```python
from build123d import *

# Parameters (mm, degrees)
F0_R     = 4
F0_R_2   = 3.1
F1_DEPTH = 22
F2_DEPTH = 27
F3_DEPTH = 5
F5_DEPTH = 25
F6_DEPTH = 25


with BuildPart() as f1:
    # F0 (on Top) → F1 (new body)
    with BuildSketch(Plane.XY):
        Circle(F0_R)
        Circle(F0_R_2, mode=Mode.SUBTRACT)
    extrude(amount=F1_DEPTH)

    # F0 (on Top) → F2 (join)
    with BuildSketch(Plane.XY):
        Circle(F0_R_2)
    extrude(amount=F2_DEPTH)

    # F0 (on Top) → F3 (join)
    with BuildSketch(Plane.XY):
        Circle(F0_R_2)
    extrude(amount=-F3_DEPTH)

    # F4 (on Right) → F5 (cut)
    with BuildSketch(Plane.YZ):
        with BuildLine():
            ThreePointArc((0, 13), (-2, 11), (0, 9))
            Line((0, 9), (0, 13))
        make_face()
        with BuildLine():
            Line((0, 13), (0, 9))
            ThreePointArc((0, 9), (1.4142135624, 9.5857864376), (2, 11))
            ThreePointArc((2, 11), (1.4142135624, 12.4142135624), (0, 13))
        make_face()
    extrude(amount=F5_DEPTH, mode=Mode.SUBTRACT)

    # F6 (cut): a face of the model
    f6_faces = [f1.faces().sort_by_distance(p)[0] for p in [
        (0, 0, 11),
    ]]
    extrude(f6_faces, amount=-F6_DEPTH, mode=Mode.SUBTRACT)


solid = f1.part
```
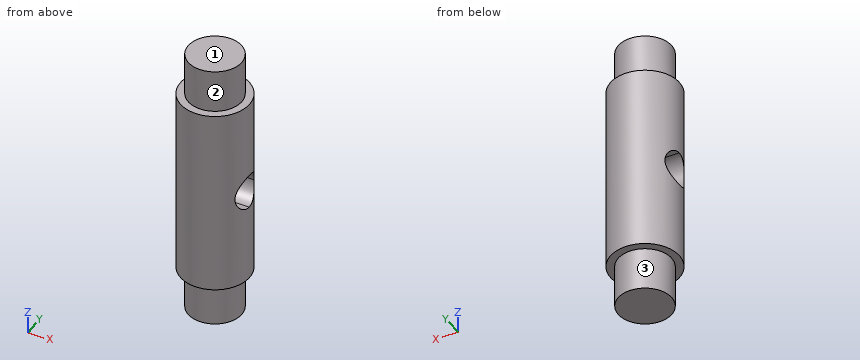
Work out the finished part from the listing and answer in its coordinate system (mm). Face numbers are marked on the shaded views. A direction names the side the tool comes from. Round coordinates to 2 decimals unless told otherwise and drop trailing zeros. Loops run counter-clockwise (first coordinate to the right, second up) from the corner with the lowest first, then second, coordinate; pieces in that order, holes last. Notation, with made-up numbers: M 69,-36.75 L 102,-36.75 A8 cw 102,-30.75 Z; hole C -31,1 d9. An arc over 180 degrees is marked long. One line per question, with ' | ' between items.
Q1. Consider line 1 along Y through (x, z) = (0, -2); line 2 along Z through (x, y) = (-2.25, 2.25); line 3 along Z through (x, y) = (0.75, 1.75). Determine where each line is inside the solid, lowest interval first. Write a range as from..to.
Conclusion:
line 1: y = -3.1..3.1 | line 2: z = 0..22 | line 3: z = -5..10.03, 11.97..27
Q2. Find section B-B, the plane y = 2.5. Give the vertices of the cut face in (x, z), then the cut area to 3 significant figures.
Conclusion:
outline: M -3.12,0 L -1.83,0 L -1.83,-5 L 1.83,-5 L 1.83,0 L 3.12,0 L 3.12,22 L 1.83,22 L 1.83,27 L -1.83,27 L -1.83,22 L -3.12,22 Z | area: 174 mm2
Q3. Find section A-A, the plane x = -2. Give the vertices of the cut face in (y, z).
Conclusion:
outline: M -3.46,0 L -2.37,0 L -2.37,-5 L 2.37,-5 L 2.37,0 L 3.46,0 L 3.46,22 L 2.37,22 L 2.37,27 L -2.37,27 L -2.37,22 L -3.46,22 Z; hole C 0,11 d4
Q4. A tool of negligible diameter and unlimited length cuts with its end or side. For the marked faces 1, 2 and 3, from which of +Z, -Z, +X, -X, +Y, -Y can it reach the whole face along a straight path? Write none if from no direction.
Conclusion:
face 1: +Z, +X, -X, +Y, -Y | face 2: +Z | face 3: -Z
Q5. Find section D-D, the plane x = 1. Give the vertices of the cut face in (y, z), then the cut area to 3 significant figures.
Conclusion:
outline: M -3.87,0 L -2.93,0 L -2.93,-5 L 2.93,-5 L 2.93,0 L 3.87,0 L 3.87,22 L 2.93,22 L 2.93,27 L -2.93,27 L -2.93,22 L -3.87,22 Z; hole C 0,11 d4 | area: 217 mm2
Q6. Each of these flat-tipped pins is pushed along its axis until it touches: pin 1 Ø1.5 at (y, z) = (-1.5, 23.5) entering from -X; pin 2 Ø1 at (y, z) = (2.5, 7.5) entering from -X. Where does it stop, or does it pass through?
Conclusion:
pin 1: stops at x = -3.01 | pin 2: stops at x = -3.46
Q7. Find section C-C, the plane z = 4.5. Give the vertices of the cut face in (x, y).
Conclusion:
outline: C 0,0 d8
